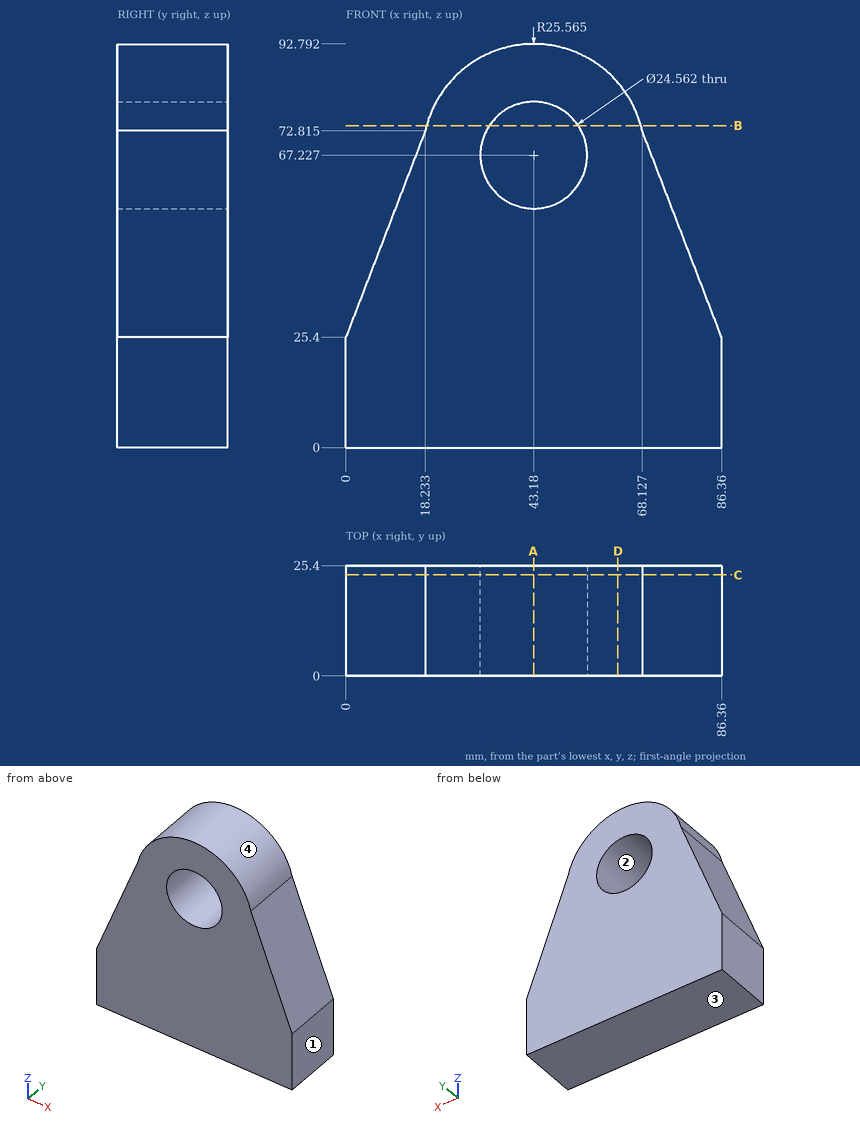
Study the drawing (mm; zero at the part's minimum x, y, z) and answer. Give positions to 0.01 mm unless a question says otherwise; leave off trailing zeros. Write each loop counter-clockwise with the first axis right and the second up, starting at its lowest first coordinate (ties: lowest second). Pieces come first, ordered by that corner, then holes. Notation, with made-up numbers: (82.25, 81) -> (133.25, 81) arc R36 cw to (133.25, 115) -> close; hole circle Ø4 at (21.25, 56). An arc over 180 degrees is marked (long way). Answer as a JSON object with one key per item and string values. Group by question number.
1) Find section D-D (x = 62.5). Write down the section's boundary in (y, z).
2) Find section C-C (y = 23.25). Write down the section's boundary in (x, z) (1 decimal), and give its area (3 significant figures).
3) This flat-tipped pin is pushed along its axis until it touches: P1, Ø10, axis at x = 48, z = 70.5, coming from the -Y side. Where does it stop, or does it pass through?
4) Find section B-B (z = 74). Write down the section's boundary in (x, y) (1 decimal), and give its area (3 significant figures).
5) Consider L1, parallel to Z at x = 43.18, y = 20.25 (1 decimal); L2, parallel to X at y = 10, z = 58.5; L3, parallel to X at y = 1, z = 73 (1 decimal). Determine where each line is inside the solid, lowest interval first. Write a range as from..to.
6) The mould has two halves that part along Z. Classify the marked faces 1, 2, 3 and 4: +Z half, -Z half, draft (parallel to the pull), parting line (faces both ways), or undercut.
7) Find section A-A (x = 43.18). Write down the section's boundary in (y, z) (1 decimal).
Values follow:
{
 "1": {"outline": "(0, 0) -> (25.4, 0) -> (25.4, 83.97) -> (0, 83.97) -> close"},
 "2": {"outline": "(0, 0) -> (86.4, 0) -> (86.4, 25.4) -> (68.1, 72.8) arc R25.6 ccw to (18.2, 72.8) -> (0, 25.4) -> close; hole circle Ø24.6 at (43.2, 67.2)", "area": "5,690 mm2"},
 "3": {"P1": "passes through"},
 "4": {"outline": "(18.5, 0) -> (32.9, 0) -> (32.9, 25.4) -> (18.5, 25.4) -> close; (53.4, 0) -> (67.8, 0) -> (67.8, 25.4) -> (53.4, 25.4) -> close", "area": "732 mm2"},
 "5": {"L1": "z = 0..54.9, 79.5..92.8", "L2": "x = 12.73..34.54, 51.82..73.63", "L3": "x = 18.3..32.3, 54..68.1"},
 "6": {"face 1": "draft", "face 2": "undercut", "face 3": "-Z half", "face 4": "+Z half"},
 "7": {"outline": "(0, 0) -> (25.4, 0) -> (25.4, 54.9) -> (0, 54.9) -> close; (0, 79.5) -> (25.4, 79.5) -> (25.4, 92.8) -> (0, 92.8) -> close"}
}
